For this review, take the finished solid that the model builds, in its own axes (mm). A direction names the side the tool comes from. Give positions to 0.01 mm unless a question says otherwise; leave off trailing zeros. Write each loop counter-clockwise with the first axis right and the second up, starting at its lowest first coordinate (ties: lowest second). Pieces come first, ordered by that corner, then holes. Notation, with made-up numbers: (-10.75, 75.25) -> (48.25, 75.25) arc R16 ccw to (48.25, 87.25) -> close; hole circle Ø11 at (-11.5, 31). An arc over 180 degrees is marked (long way). Write item = value, one per line.
```python
from build123d import *


with BuildPart() as part:
    # Balayage1: sweep along a path in Esquisse1
    with BuildLine(Plane.XY) as balayage1_path:
        Line((86.98, 39.930935376), (-3.41, 10.458102122))
        ThreePointArc((-3.41, 10.458102122), (-11, 0), (-3.41, -10.458102122))
        Line((-3.41, -10.458102122), (86.98, -39.930935376))
        ThreePointArc((86.98, -39.930935376), (142, 0), (86.98, 39.930935376))
    # Esquisse2 → Balayage1 (sweep)
    with BuildSketch(Plane(origin=(0, 0, 0), x_dir=(1, 0, 0), z_dir=(0, 1, 0))):
        Polygon((-13.5, -3), (-13.5, 3), (-11, 0.5), (-11, -0.5), align=None)
    sweep(path=balayage1_path.line)


solid = part.part
```
(1) For pin 1 (1.5 mm diameter, centred on x = 79.5, z = 2.5, fed in from +Y), flat-tipped, find the tip position at first contact; note if it passes through.
Answers below:
pin_1 = 40.37
(2) Tool access review of faces 1 (the face through (-11.12, 0.2, 0.62)), 2 (the face through (42.42, -25.4, 0.01)), 3 (the face through (42.04, -26.57, -1.73)): name each direction out of +Z, -Z, +X, -X, +Y, -Y from which nothing blocks a thin tool from reaching the whole face with its end or side.
Answers below:
face_1 = +Z
face_2 = +Z, -Z
face_3 = -Z
(3) Take a section at B-B (x = 100). Write out the cut boundary in (y, z), plus the area to 3 significant figures.
Answers below:
outline = (-44.5, -3) -> (-42, -0.5) -> (-42, 0.5) -> (-44.5, 3) -> close; (42, -0.5) -> (44.5, -3) -> (44.5, 3) -> (42, 0.5) -> close
area = 17.5 mm^2
(4) To check wall thickness, follow probe 1 along Y at (x, z) = (100, -0.1); probe 2 along X at (y, z) = (1.5, -0.25); probe 3 along Y at (x, z) = (115.5, 2). State the ranges of each line that lie inside material, in increasing order.
Answers below:
probe_1 = -44.5 to -42, 42 to 44.5
probe_2 = -13.42 to -10.9, 141.97 to 144.47
probe_3 = -41.71 to -40.64, 40.64 to 41.71
(5) The part is to be moulded in two halves that separate along X. For faces 4 (the face through (144.484, -1.175, 0.042)), 5 (the face through (-13.5, 0.2, 0)), 6 (the face through (142.107, -1.112, 0.621)), say which applies: released by +X, released by -X, zero draft, split by the parting line, or undercut.
Answers below:
face_4 = split by the parting line
face_5 = released by -X
face_6 = undercut
(6) Take a section at A-A (y = 0). Write out the cut boundary in (x, z), plus the area to 3 significant figures.
Answers below:
outline = (-13.5, -3) -> (-11, -0.5) -> (-11, 0.5) -> (-13.5, 3) -> close; (142, -0.5) -> (144.5, -3) -> (144.5, 3) -> (142, 0.5) -> close
area = 17.5 mm^2
